Verification items for this drawing (mm, ordinates from the low corner). A direction names the side the tool comes from. Round coordinates to 2 decimals unless told otherwise and drop trailing zeros. Loops run counter-clockwise (first coordinate to the right, second up) from the corner with the lowest first, then second, coordinate; pieces in that order, holes last. Notation, with made-up numbers: M -2,40 L 18,40 A17 ccw 18,52 Z; hole C -1,34 d8. An arc over 180 degrees is marked long. Write item = value, one per line. Start each with the question number.
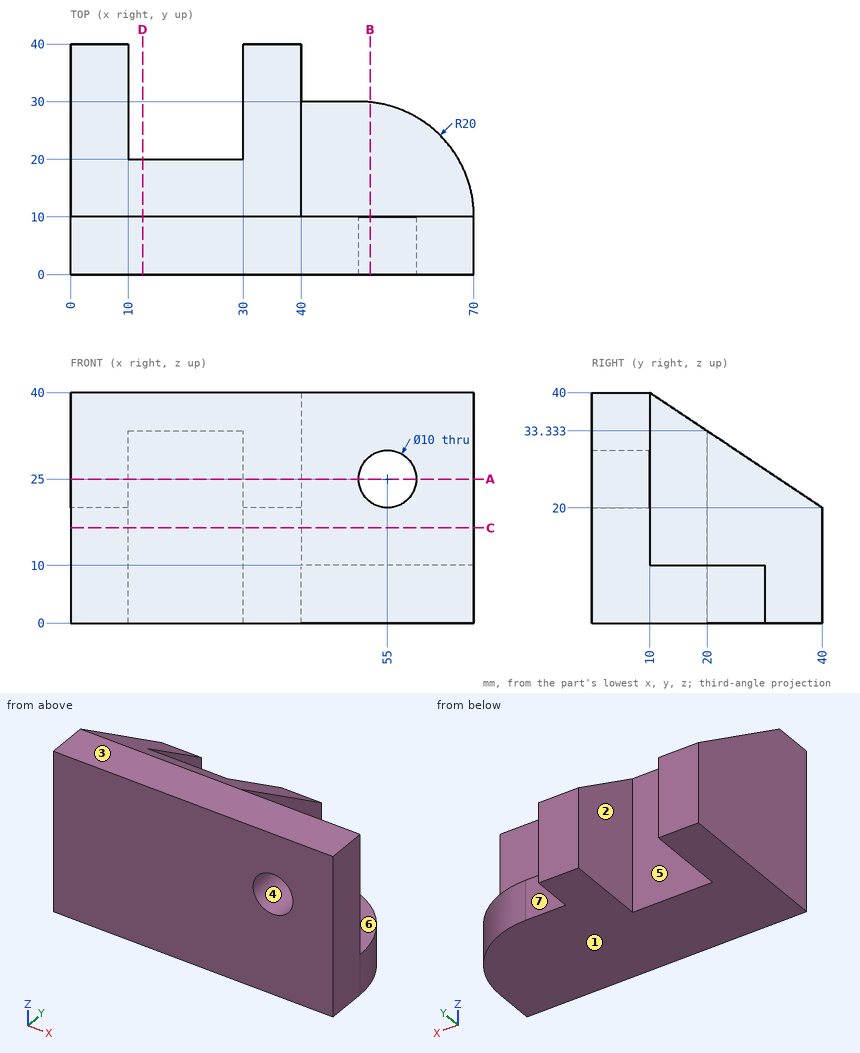
1. Gauge pin test, flat ends, axial feed: P1, Ø3, axis at y = 35, z = 13.5, coming from the +X side; P2, Ø5, axis at x = 58.5, z = 25, coming from the +Y side; P3, Ø8, axis at x = 47, z = 4, coming from the +Y side; P4, Ø9, axis at x = 55, z = 25, coming from the -Y side. Record the tip position at first contact, or that the pin passes through.
2. Section check A-A, the plane z = 25. Enter the section's corners in (x, y), and give its area (3 significant figures).
3. Tool access check on the marked faces 5, 6 and 7. Record the directions out of +Z, -Z, +X, -X, +Y, -Y that give a thin tool (end or side, any length) a straight path to the whole face; none if there is none.
4. Section check D-D, the plane x = 12.5. Enter the section's corners in (y, z).
5. Section check C-C, the plane z = 16.5. Enter the section's corners in (x, y), and give its area (3 significant figures).
6. Section check B-B, the plane x = 52. Enter the section's corners in (y, z), and give its area (3 significant figures).
7. Mould release check, pull along Z, two halves, no side actions. Record for the marked faces 1, 2, 3 and 4: pulls with the +Z half, pulls with the -Z half, needs draft (parallel to the pull), parting line crosses it, or undercut.
8. Thickness scan on line 1 (Z direction, x = 55, y = 4); line 2 (X direction, y = 4.75, z = 25); line 3 (X direction, y = 29.5, z = 21). Record the ranges inside material, lowest first.
Computed values:
q1.P1 = 40
q1.P2 = 10
q1.P3 = 30
q1.P4 = through
q2.outline = M 0,0 L 50,0 L 50,10 L 40,10 L 40,32.5 L 30,32.5 L 30,20 L 10,20 L 10,32.5 L 0,32.5 Z; M 60,0 L 70,0 L 70,10 L 60,10 Z
q2.area = 1,250 mm2
q3.face_5 = +Z, -Z, +Y
q3.face_6 = +Z, +X, +Y
q3.face_7 = +Z, -Z, +X, +Y
q4.outline = M 0,0 L 20,0 L 20,33.33 L 10,40 L 0,40 Z
q5.outline = M 0,0 L 70,0 L 70,10 L 40,10 L 40,40 L 30,40 L 30,20 L 10,20 L 10,40 L 0,40 Z
q5.area = 1,500 mm2
q6.outline = M 0,0 L 29.9,0 L 29.9,10 L 10,10 L 10,21 L 0,21 Z; M 0,29 L 10,29 L 10,40 L 0,40 Z
q6.area = 519 mm2
q7.face_1 = pulls with the -Z half
q7.face_2 = needs draft
q7.face_3 = pulls with the +Z half
q7.face_4 = undercut
q8.line_1 = 0 to 20, 30 to 40
q8.line_2 = 0 to 50, 60 to 70
q8.line_3 = 0 to 10, 30 to 40
